The listing builds one solid part. Answer for the finished solid, in the listing's coordinates (mm). Give positions to 0.01 mm unless a question says otherwise; leave off trailing zeros. Order: outer loops, then holes, each group sorted by start corner. A loop starts at its lowest first (then second) coordinate and runs counter-clockwise, first axis right, second up. Notation, with made-up numbers: (6, 30) -> (53, 30) arc R15 ccw to (53, 55) -> close; hole circle Ø6 at (-28, -20). An arc over 180 degrees is marked (long way). Answer as a JSON object with one key per item and string values. Group by question number.
```python
from build123d import *

# Parameters (mm, degrees)
BOSS_EXTRUDE1_DEPTH = 3
SKETCH2_W           = 3
SKETCH2_H           = 15
CUT_EXTRUDE1_DEPTH  = 10
CUT_EXTRUDE5_DEPTH  = 10


with BuildPart() as part:
    # Sketch1 → Boss-Extrude1 (new body)
    with BuildSketch(Plane.XY):
        Polygon((75, 45), (-75, 45), (-75, 25), (-78, 25), (-78, 10), (-75, 10), (-75, -10), (-78, -10), (-78, -25), (-75, -25), (-75, -45), (-50, -45), (-50, -48), (-35, -48), (-35, -45), (35, -45), (35, -48), (50, -48), (50, -45), (75, -45), (75, -25), (78, -25), (78, -10), (75, -10), (75, 10), (78, 10), (78, 25), (75, 25), align=None)
    extrude(amount=BOSS_EXTRUDE1_DEPTH)

    # Sketch2 → Cut-Extrude1 (cut)
    with BuildSketch(Plane.XY.offset(3)):
        Rectangle(SKETCH2_W, SKETCH2_H)
    extrude(amount=-CUT_EXTRUDE1_DEPTH, mode=Mode.SUBTRACT)

    # Sketch6 → Cut-Extrude5 (cut)
    with BuildSketch(Plane.XY.offset(3)):
        with BuildLine():
            Line((5.290512726, 25.935056248), (2.295363862, 16.311934545))
            Line((2.295363862, 16.311934545), (-2.295363862, 16.311934545))
            Line((-2.295363862, 16.311934545), (-5.290512726, 25.935056248))
            Line((-5.290512726, 25.935056248), (-5.287204108, 13.065687756))
            Line((-5.287204108, 13.065687756), (-4.373165869, 13.065687756))
            ThreePointArc((-4.373165869, 13.065687756), (-3.915305203, 13.527588879), (-3.287366333, 13.696945937))
            Line((-3.287366333, 13.696945937), (-3.287524442, 14.311934545))
            Line((-3.287524442, 14.311934545), (3.287524442, 14.311934545))
            Line((3.287524442, 14.311934545), (3.287366333, 13.696945937))
            ThreePointArc((3.287366333, 13.696945937), (3.915305203, 13.527588879), (4.373165869, 13.065687756))
            Line((4.373165869, 13.065687756), (5.287204108, 13.065687756))
            Line((5.287204108, 13.065687756), (5.290512726, 25.935056248))
        make_face()
        with BuildLine():
            Line((5.285908962, 8.028025182), (5.2868631, 11.739287))
            Line((5.2868631, 11.739287), (4.317442352, 11.739287))
            ThreePointArc((4.317442352, 11.739287), (3.869108183, 11.340735142), (3.286723602, 11.19694602))
            Line((3.286723602, 11.19694602), (3.285909029, 8.028539367))
            ThreePointArc((3.285909029, 8.028539367), (3.374432245, 6.505542997), (3.639582158, 5.003194892))
            ThreePointArc((3.639582158, 5.003194892), (6.055992917, 1.239562801), (10.295107821, -0.186576152))
            ThreePointArc((10.295107821, -0.186576152), (11.01438813, -0.194494412), (11.732516685, -0.153042755))
            ThreePointArc((11.732516685, -0.153042755), (18.692972821, 4.404939535), (18.821664118, 12.723989405))
            ThreePointArc((18.821664118, 12.723989405), (25.37715821, 12.9694755), (31.476327164, 10.553920845))
            ThreePointArc((31.476327164, 10.553920845), (37.518458896, -5.149561028), (24.647485484, -15.98675357))
            ThreePointArc((24.647485484, -15.98675357), (24.695354215, -15.831004559), (24.740416096, -15.674420407))
            ThreePointArc((24.740416096, -15.674420407), (24.374260224, -11.19523634), (21.190905903, -8.022947688))
            ThreePointArc((21.190905903, -8.022947688), (16.646624705, -7.250909085), (12.327665086, -8.861226761))
            ThreePointArc((12.327665086, -8.861226761), (10.583620787, -7.776302438), (8.564637884, -7.398864573))
            ThreePointArc((8.564637884, -7.398864573), (5.000034739, -8.19121848), (2.10219111, -10.413092149))
            ThreePointArc((2.10219111, -10.413092149), (0.980226646, -11.88188736), (0, -13.448833229))
            ThreePointArc((0, -13.448833229), (-0.980226646, -11.88188736), (-2.10219111, -10.413092149))
            ThreePointArc((-2.10219111, -10.413092149), (-5.000034739, -8.19121848), (-8.564637884, -7.398864573))
            ThreePointArc((-8.564637884, -7.398864573), (-10.583620787, -7.776302438), (-12.327665086, -8.861226761))
            ThreePointArc((-12.327665086, -8.861226761), (-16.646624705, -7.250909085), (-21.190905903, -8.022947688))
            ThreePointArc((-21.190905903, -8.022947688), (-24.374260224, -11.19523634), (-24.740416096, -15.674420407))
            ThreePointArc((-24.740416096, -15.674420407), (-24.695354215, -15.831004559), (-24.647485484, -15.98675357))
            ThreePointArc((-24.647485484, -15.98675357), (-37.518458896, -5.149561028), (-31.476327164, 10.553920845))
            ThreePointArc((-31.476327164, 10.553920845), (-25.37715821, 12.9694755), (-18.821664118, 12.723989405))
            ThreePointArc((-18.821664118, 12.723989405), (-18.692972821, 4.404939535), (-11.732516685, -0.153042755))
            ThreePointArc((-11.732516685, -0.153042755), (-11.01438813, -0.194494412), (-10.295107821, -0.186576152))
            ThreePointArc((-10.295107821, -0.186576152), (-6.055992917, 1.239562801), (-3.639582158, 5.003194892))
            ThreePointArc((-3.639582158, 5.003194892), (-3.374432245, 6.505542997), (-3.285909029, 8.028539367))
            Line((-3.285909029, 8.028539367), (-3.286723602, 11.19694602))
            ThreePointArc((-3.286723602, 11.19694602), (-3.869108183, 11.340735142), (-4.317442352, 11.739287))
            Line((-4.317442352, 11.739287), (-5.2868631, 11.739287))
            Line((-5.2868631, 11.739287), (-5.285908962, 8.028025182))
            ThreePointArc((-5.285908962, 8.028025182), (-5.360904336, 6.737768387), (-5.585534863, 5.465004453))
            ThreePointArc((-5.585534863, 5.465004453), (-7.308177113, 2.799425217), (-10.325195997, 1.814333325))
            ThreePointArc((-10.325195997, 1.814333325), (-10.937431926, 1.804308669), (-11.548794517, 1.838500909))
            ThreePointArc((-11.548794517, 1.838500909), (-17.428845514, 6.476374098), (-15.585134149, 13.734858501))
            ThreePointArc((-15.585134149, 13.734858501), (-24.273750539, 15.128136766), (-32.579650708, 12.222056678))
            ThreePointArc((-32.579650708, 12.222056678), (-38.93241703, -7.310810177), (-21.328283314, -17.893106884))
            ThreePointArc((-21.328283314, -17.893106884), (-22.225314868, -16.599112533), (-22.8135279, -15.138601519))
            ThreePointArc((-22.8135279, -15.138601519), (-22.559974367, -12.036881652), (-20.355583301, -9.840153276))
            ThreePointArc((-20.355583301, -9.840153276), (-15.796843839, -9.421233335), (-11.984787413, -11.956154477))
            ThreePointArc((-11.984787413, -11.956154477), (-10.701852428, -10.107966912), (-8.56669627, -9.398863514))
            ThreePointArc((-8.56669627, -9.398863514), (-5.845441544, -10.003754641), (-3.633197893, -11.699955866))
            ThreePointArc((-3.633197893, -11.699955866), (-1.414932414, -15.040464669), (0, -18.7924864))
            ThreePointArc((0, -18.7924864), (1.414932414, -15.040464669), (3.633197893, -11.699955866))
            ThreePointArc((3.633197893, -11.699955866), (5.845441544, -10.003754641), (8.56669627, -9.398863514))
            ThreePointArc((8.56669627, -9.398863514), (10.701852428, -10.107966912), (11.984787413, -11.956154477))
            ThreePointArc((11.984787413, -11.956154477), (15.796843839, -9.421233335), (20.355583301, -9.840153276))
            ThreePointArc((20.355583301, -9.840153276), (22.559974367, -12.036881652), (22.8135279, -15.138601519))
            ThreePointArc((22.8135279, -15.138601519), (22.225314868, -16.599112533), (21.328283314, -17.893106884))
            ThreePointArc((21.328283314, -17.893106884), (38.93241703, -7.310810177), (32.579650708, 12.222056678))
            ThreePointArc((32.579650708, 12.222056678), (24.273750539, 15.128136766), (15.585134149, 13.734858501))
            ThreePointArc((15.585134149, 13.734858501), (17.428845514, 6.476374098), (11.548794517, 1.838500909))
            ThreePointArc((11.548794517, 1.838500909), (10.937431926, 1.804308669), (10.325195997, 1.814333325))
            ThreePointArc((10.325195997, 1.814333325), (7.308177113, 2.799425217), (5.585534863, 5.465004453))
            ThreePointArc((5.585534863, 5.465004453), (5.360904336, 6.737768387), (5.285908962, 8.028025182))
        make_face()
    extrude(amount=-CUT_EXTRUDE5_DEPTH, mode=Mode.SUBTRACT)


solid = part.part
```
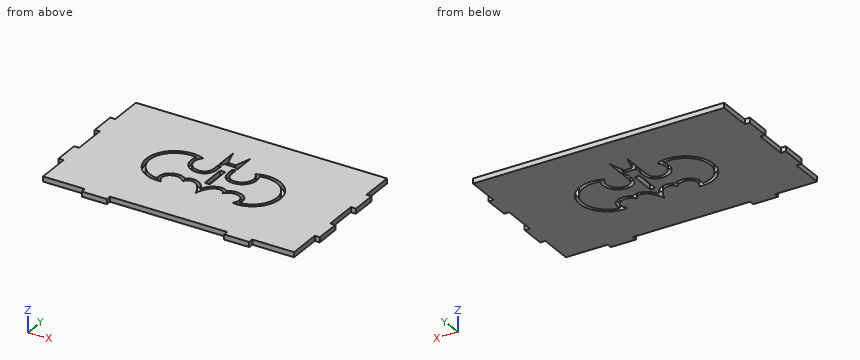
(1) Find the intervals of material crossed by line 1 along Y through (x, z) = (-8.5, 1); line 2 along Y through (x, z) = (-31.5, 1.15); line 3 along X through (y, z) = (-4, 1.35) (3 decimals), in increasing order. Write a range as [from, to].
(2) A cutting plane is placed at B-B (y = 3.5). State how many separate pieces and enclosed holes the cut face has, and give its area (3 significant figures).
(3) Flat-ended cylindrical pins translate along their axes: pin 1 Ø1.5 at (x, z) = (-76.5, 1.5) entering from +Y; pin 2 Ø1 at (y, z) = (-34, 1) entering from -X; pin 3 Ø0.8 at (x, z) = (5, 1.5) entering from -Y. Find the tip coordinate at first contact, or state that the pin passes through.
(4) A cutting plane is placed at A-A (y = 21.5). Determine the outline of the cut face in (x, z).
(5) A cutting plane is placed at D-D (x = 51.5). Determine the outline of the cut face in (y, z), and give its area (3 significant figures).
Check sheet entries:
{
 "1": {"line 1": "y = [-45, -9.4], [-7.4, 0.03], [2.13, 45]", "line 2": "y = [-45, -15.95], [-13.61, 10.54], [12.88, 45]", "line 3": "x = [-75, -39.791], [-37.765, -1.5], [1.5, 37.765], [39.791, 75]"},
 "2": {"separate pieces": "8", "enclosed holes": "0", "area": "398 mm2"},
 "3": {"pin 1": "stops at y = 25", "pin 2": "stops at x = -75", "pin 3": "stops at y = -45"},
 "4": {"outline": "(-78, 0) -> (-5.29, 0) -> (-5.29, 3) -> (-78, 3) -> close; (-3.91, 0) -> (3.91, 0) -> (3.91, 3) -> (-3.91, 3) -> close; (5.29, 0) -> (78, 0) -> (78, 3) -> (5.29, 3) -> close"},
 "5": {"outline": "(-45, 0) -> (45, 0) -> (45, 3) -> (-45, 3) -> close", "area": "270 mm2"}
}
